Answer from the drawing. Dimensions are ordinates in mm from the lowest x, y and z of the part. A direction names the side the tool comes from. Round coordinates to 2 decimals unless told otherwise and drop trailing zeros. Loops run counter-clockwise (first coordinate to the right, second up) from the corner with the lowest first, then second, coordinate; pieces in that order, holes last. Notation, with made-up numbers: (-21, 5) - (-6, 5) arc R29 cw to (-6, 33) - close; hole circle Ø7 at (-6, 23.5). An arc over 180 degrees is marked (long way). Return JSON: item names as keys, results as strings.
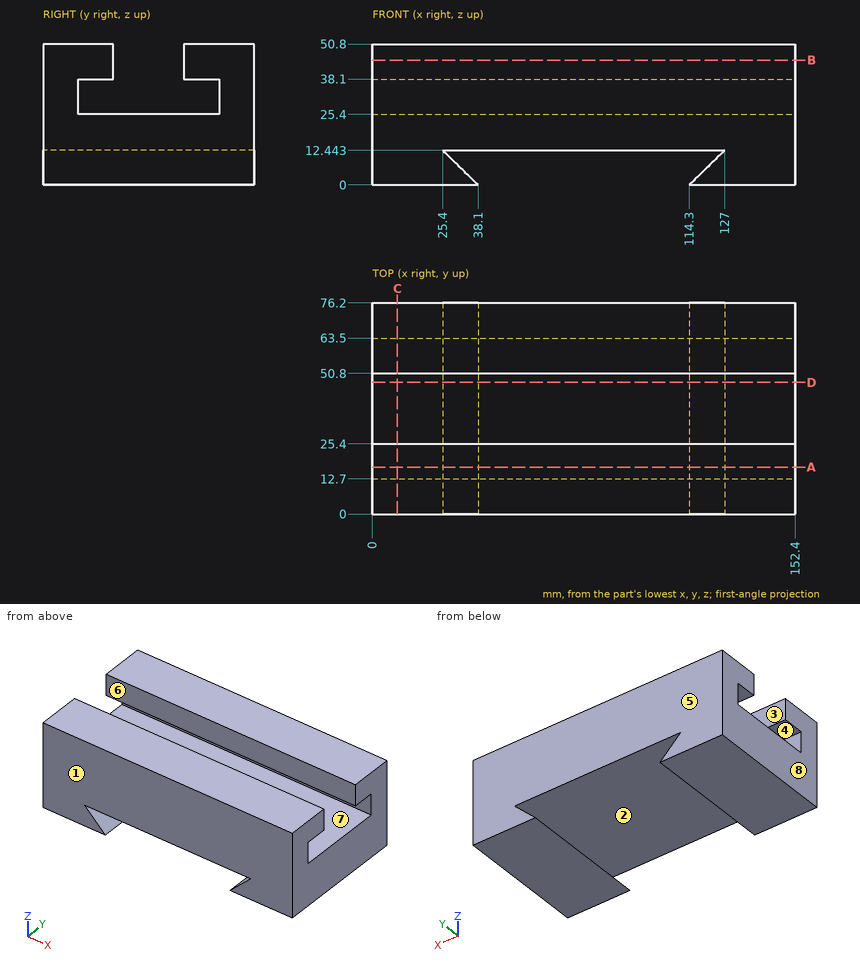
1) A tool of negligible diameter and unlimited length cuts with its end or side. For the marked faces 1, 2, 3 and 4, from which of +Z, -Z, +X, -X, +Y, -Y can it reach the whole face along a straight path? Write none if from no direction.
Verdict:
{"face 1": "+Z, -Z, +X, -X, -Y", "face 2": "+Y, -Y", "face 3": "+Z, +X, -X", "face 4": "+X, -X"}
2) Find the intervals of material crossed by L1, parallel to Y at x = 60.5, z = 41; L2, parallel to Z at x = 102, y = 54; L3, parallel to Y at x = 131, z = 30.5, in increasing order.
Verdict:
{"L1": "y = 0 to 25.4, 50.8 to 76.2", "L2": "z = 12.44 to 25.4, 38.1 to 50.8", "L3": "y = 0 to 12.7, 63.5 to 76.2"}
3) Section C-C (x = 9) is taken. Give the vertices of the cut face in (y, z), and give its area (3 significant figures).
Verdict:
{"outline": "(0, 0) - (76.2, 0) - (76.2, 50.8) - (50.8, 50.8) - (50.8, 38.1) - (63.5, 38.1) - (63.5, 25.4) - (12.7, 25.4) - (12.7, 38.1) - (25.4, 38.1) - (25.4, 50.8) - (0, 50.8) - close", "area": "2,900 mm2"}
4) Section D-D (y = 47.5) is taken. Give the vertices of the cut face in (x, z).
Verdict:
{"outline": "(0, 0) - (38.1, 0) - (25.4, 12.44) - (127, 12.44) - (114.3, 0) - (152.4, 0) - (152.4, 25.4) - (0, 25.4) - close"}
5) A flat-ended cylindrical pin translates along its axis: pin 1 (1 mm diameter, centred on x = 102, y = 45.5, fed in from -Z). Find the tip coordinate at first contact, or state that the pin passes through.
Verdict:
{"pin 1": "stops at z = 12.44"}
6) Section B-B (z = 45) is taken. Give the vertices of the cut face in (x, y), and give its area (3 significant figures).
Verdict:
{"outline": "(0, 0) - (152.4, 0) - (152.4, 25.4) - (0, 25.4) - close; (0, 50.8) - (152.4, 50.8) - (152.4, 76.2) - (0, 76.2) - close", "area": "7,740 mm2"}
7) Determine the mould class of the marked faces 5, 6, 7 and 8 for opening direction Y: pulls with the +Y half, pulls with the -Y half, needs draft (parallel to the pull), parting line crosses it, or undercut.
Verdict:
{"face 5": "pulls with the +Y half", "face 6": "undercut", "face 7": "undercut", "face 8": "needs draft"}
8) Section A-A (y = 17) is taken. Give the vertices of the cut face in (x, z), and give its area (3 significant figures).
Verdict:
{"outline": "(0, 0) - (38.1, 0) - (25.4, 12.44) - (127, 12.44) - (114.3, 0) - (152.4, 0) - (152.4, 25.4) - (0, 25.4) - close; (0, 38.1) - (152.4, 38.1) - (152.4, 50.8) - (0, 50.8) - close", "area": "4,700 mm2"}
